Here's how the part is built. I have some questions about the finished solid (model axes, mm). A direction names the side the tool comes from. Round coordinates to 2 decimals unless told otherwise and drop trailing zeros. Write each loop counter-clockwise with the first axis right and the second up, starting at its lowest first coordinate (ties: lowest second). Pieces come first, ordered by that corner, then holes. Notation, with made-up numbers: (39.25, -20) - (61.25, -20) arc R18 ccw to (61.25, -13) - close; hole circle Ø9 at (32, 64.5). An arc over 180 degrees is marked (long way). One line per item, written item: value. Start each with the question number.
Item 1: Imagine slicing it at D-D, the plane x = -2. Please give me the cut outline in (y, z), then the cut area to 3 significant figures.
Item 2: Imagine slicing it at B-B, the plane x = 0. Please give me the cut outline in (y, z).
Item 3: Imagine slicing it at A-A, the plane z = 0. Please give me the cut outline in (x, y).
Item 4: Imagine slicing it at C-C, the plane y = 8.5. Please give me the cut outline in (x, z).
Item 5: For P1, Ø2, axis at x = -1.5, z = -2.5, coming from the +Y side; P2, Ø1, axis at y = 3, z = 2.5, coming from the -X side; P3, Ø4, axis at x = -3, y = 3, coming from the -Z side, each with a flat end and sliding along its axis, tell me the tip position at first contact or that it passes through.
Item 6: If I drill on line 1 (Y direction, x = -2, z = -2.75); line 2 (Z direction, x = 0, y = 8.25); line 3 (Y direction, x = 0.25, z = -2), over which ranges is the centre line in solid material (lowest first)?
Item 7: For faces 1 (the face through (-3.746, 1.849, -0.165)), 2 (the face through (2, 7.75, 1)), which set-ups out of +Z, -Z, +X, -X, +Y, -Y let a thin tool reach every point of the face, with its end or its side?
```python
from build123d import *

# Parameters (mm, degrees)
SKETCH1_R           = 3.75
BOSS_EXTRUDE1_DEPTH = 7.75
SKETCH2_R           = 3.75
SKETCH2_R_2         = 2.5
CUT_EXTRUDE1_DEPTH  = 4
SKETCH3_R           = 1.65
BOSS_EXTRUDE2_DEPTH = 2


with BuildPart() as part:
    # Sketch1 → Boss-Extrude1 (new body)
    with BuildSketch(Plane(origin=(0, 0, 0), x_dir=(1, 0, 0), z_dir=(0, 1, 0))):
        Circle(SKETCH1_R)
    extrude(amount=BOSS_EXTRUDE1_DEPTH)

    # Sketch2 → Cut-Extrude1 (cut)
    with BuildSketch(Plane(origin=(0, 7.75, 0), x_dir=(1, 0, 0), z_dir=(0, 1, 0))):
        Circle(SKETCH2_R)
        Circle(SKETCH2_R_2, mode=Mode.SUBTRACT)
    extrude(amount=-CUT_EXTRUDE1_DEPTH, mode=Mode.SUBTRACT)

    # Sketch3 → Boss-Extrude2 (add)
    with BuildSketch(Plane(origin=(0, 7.75, 0), x_dir=(1, 0, 0), z_dir=(0, 1, 0))):
        Circle(SKETCH3_R)
    extrude(amount=BOSS_EXTRUDE2_DEPTH)


solid = part.part
```
Values follow:
1. outline: (0, -3.17) - (3.75, -3.17) - (3.75, -1.5) - (7.75, -1.5) - (7.75, 1.5) - (3.75, 1.5) - (3.75, 3.17) - (0, 3.17) - close
1. area: 35.8 mm^2
2. outline: (0, -3.75) - (3.75, -3.75) - (3.75, -2.5) - (7.75, -2.5) - (7.75, -1.65) - (9.75, -1.65) - (9.75, 1.65) - (7.75, 1.65) - (7.75, 2.5) - (3.75, 2.5) - (3.75, 3.75) - (0, 3.75) - close
3. outline: (-3.75, 0) - (3.75, 0) - (3.75, 3.75) - (2.5, 3.75) - (2.5, 7.75) - (1.65, 7.75) - (1.65, 9.75) - (-1.65, 9.75) - (-1.65, 7.75) - (-2.5, 7.75) - (-2.5, 3.75) - (-3.75, 3.75) - close
4. outline: circle Ø3.3 at (0, 0)
5. P1: stops at y = 7.75
5. P2: stops at x = -3.17
5. P3: stops at z = -3.61
6. line 1: y = 0 to 3.75
6. line 2: z = -1.65 to 1.65
6. line 3: y = 0 to 7.75
7. face 1: +Y, -Y
7. face 2: +Y
